```python
from build123d import *

# Parameters (mm, degrees)
SKETCH1_R             = 24.75
SKETCH1_R_2           = 21.75
BOSS_EXTRUDE1_DEPTH   = 90
BOSS_EXTRUDE3_START   = 72
SKETCH5_R             = 29.75
SKETCH5_R_2           = 21.75
BOSS_EXTRUDE3_DEPTH   = 5
SKETCH7_R             = 24.75
SKETCH7_R_2           = 21.75
BOSS_EXTRUDE4_DEPTH   = 2.5
BOSS_EXTRUDE5_START   = -5
SKETCH6_R             = 2
BOSS_EXTRUDE5_DEPTH   = 5
MIRROR2_START         = -92.5
MIRROR2_OUTLINE_R     = 24.75
MIRROR2_OUTLINE_R_2   = 21.75
MIRROR2_DEPTH         = 92.5
MIRROR2_START_2       = 67
MIRROR2_2_OUTLINE_R   = 29.75
MIRROR2_2_OUTLINE_R_2 = 24.75
MIRROR2_2_DEPTH       = 5
MIRROR2_3_OUTLINE_R   = 2
MIRROR2_3_DEPTH       = 5


# Read off the part's stored shape, not the designer's step: Mirror2
with BuildPart() as part:
    # Sketch1 → Boss-Extrude1 (new body)
    with BuildSketch(Plane.XY):
        with Locations(Location((0, 0, 0), (0, 0, 180))):
            Circle(SKETCH1_R)
        with Locations(Location((0, 0, 0), (0, 0, 180))):
            Circle(SKETCH1_R_2, mode=Mode.SUBTRACT)
    extrude(amount=BOSS_EXTRUDE1_DEPTH)

    # Sketch5 → Boss-Extrude3 (add)
    with BuildSketch(Plane.XY.offset(BOSS_EXTRUDE3_START)):
        Circle(SKETCH5_R)
        with Locations(Location((0, 0, 0), (0, 0, 180))):
            Circle(SKETCH5_R_2, mode=Mode.SUBTRACT)
    extrude(amount=BOSS_EXTRUDE3_DEPTH)

    # Sketch7 → Boss-Extrude4 (add, symmetric)
    with BuildSketch(Plane.XY.offset(90)):
        with Locations(Location((0, 0, 0), (0, 0, 180))):
            Circle(SKETCH7_R)
        with Locations(Location((0, 0, 0), (0, 0, 180))):
            Circle(SKETCH7_R_2, mode=Mode.SUBTRACT)
    extrude(amount=BOSS_EXTRUDE4_DEPTH, both=True)

    # Sketch6 → Boss-Extrude5 (add)
    with BuildSketch(Plane.XY.offset(92.5).offset(BOSS_EXTRUDE5_START)):
        with BuildLine():
            Line((-22.997666259, 9.147122314), (-33.267406372, 22.947582732))
            Line((-33.267406372, 22.947582732), (-22.947582732, 33.267406372))
            Line((-22.947582732, 33.267406372), (-9.147122314, 22.997666259))
            ThreePointArc((-9.147122314, 22.997666259), (-17.500892834, 17.500892834), (-22.997666259, 9.147122314))
        make_face()
        with Locations((-20.04683438, 22.097086912)):
            Circle(SKETCH6_R, mode=Mode.SUBTRACT)
        with Locations((-27.04683438, 22.097086912)):
            Circle(SKETCH6_R, mode=Mode.SUBTRACT)
    boss_extrude5 = extrude(amount=BOSS_EXTRUDE5_DEPTH)

    # Mirror1: Boss-Extrude5 across plane
    add(boss_extrude5.mirror(Plane(origin=(0, 0, 0), x_dir=(0, 0, 1), z_dir=(1, 0, 0))))

    # Mirror2 outline → Mirror2 (add)
    with BuildSketch(Plane.XY.offset(MIRROR2_START)):
        Circle(MIRROR2_OUTLINE_R)
        Circle(MIRROR2_OUTLINE_R_2, mode=Mode.SUBTRACT)
    extrude(amount=MIRROR2_DEPTH)

    # Mirror2 2 outline → Mirror2 2 (add)
    with BuildSketch(Plane.XY.offset(MIRROR2_START_2)):
        Circle(MIRROR2_2_OUTLINE_R)
        Circle(MIRROR2_2_OUTLINE_R_2, mode=Mode.SUBTRACT)
    extrude(amount=MIRROR2_2_DEPTH)

    # Mirror2 3 outline → Mirror2 3 (add)
    # profile 1 of 2: a face of its own
    with BuildSketch(Plane.XY.offset(MIRROR2_START)):
        with BuildLine():
            ThreePointArc((9.147122314, 22.997666259), (17.500892834, 17.500892834), (22.997666259, 9.147122314))
            Line((22.997666259, 9.147122314), (33.267406372, 22.947582732))
            Line((33.267406372, 22.947582732), (22.947582732, 33.267406372))
            Line((22.947582732, 33.267406372), (9.147122314, 22.997666259))
        make_face()
        with Locations((20.04683438, 22.097086912)):
            Circle(MIRROR2_3_OUTLINE_R, mode=Mode.SUBTRACT)
        with Locations((27.04683438, 22.097086912)):
            Circle(MIRROR2_3_OUTLINE_R, mode=Mode.SUBTRACT)
    # profile 2 of 2: a face of its own
    with BuildSketch(Plane.XY.offset(MIRROR2_START)):
        with BuildLine():
            ThreePointArc((-22.997666259, 9.147122314), (-17.500892834, 17.500892834), (-9.147122314, 22.997666259))
            Line((-9.147122314, 22.997666259), (-22.947582732, 33.267406372))
            Line((-22.947582732, 33.267406372), (-33.267406372, 22.947582732))
            Line((-33.267406372, 22.947582732), (-22.997666259, 9.147122314))
        make_face()
        with Locations((-20.04683438, 22.097086912)):
            Circle(MIRROR2_3_OUTLINE_R, mode=Mode.SUBTRACT)
        with Locations((-27.04683438, 22.097086912)):
            Circle(MIRROR2_3_OUTLINE_R, mode=Mode.SUBTRACT)
    extrude(amount=MIRROR2_3_DEPTH)


solid = part.part
```
Input: part model. Units: mm. Frame: model coordinates. A direction names the side the tool comes from. Coordinates: 2 decimals unless noted, no trailing zeros. Write each loop counter-clockwise with the first axis right and the second up, starting at its lowest first coordinate (ties: lowest second). Pieces come first, ordered by that corner, then holes. Notation, with made-up numbers: (37.5, -9) -> (52.5, -9) arc R26 cw to (52.5, 15) -> close; hole circle Ø6 at (68.5, 80). An arc over 180 degrees is marked (long way). Answer as a JSON object with one key per item and string values.
1. Section A-A on x = 0. Return the cut outline in (y, z).
Result set:
{"outline": "(-29.75, 67) -> (-24.75, 67) -> (-24.75, -92.5) -> (-21.75, -92.5) -> (-21.75, 92.5) -> (-24.75, 92.5) -> (-24.75, 77) -> (-29.75, 77) -> close; (21.75, -92.5) -> (24.75, -92.5) -> (24.75, 67) -> (29.75, 67) -> (29.75, 77) -> (24.75, 77) -> (24.75, 92.5) -> (21.75, 92.5) -> close"}
2. Section C-C on z = 62. Return the cut outline in (x, y), then the cut area to 3 significant figures.
Result set:
{"outline": "circle Ø49.5 at (0, 0); hole circle Ø43.5 at (0, 0)", "area": "438 mm2"}
3. Mould query, pull axis Y, two halves, no side actions, for faces 5 (the face through (25.05, 22.19, -90.04)), 6 (the face through (-28.18, 28.035, 89.965)), 7 (the face through (24, 21, 87.5)). Classes: released by +Y, released by -Y, zero draft, split by the parting line, or undercut.
Result set:
{"face 5": "undercut", "face 6": "released by +Y", "face 7": "zero draft"}
4. Material intervals for line 1 (Y direction, x = -12.5, z = -34); line 2 (Y direction, x = -11, z = 18); line 3 (X direction, y = 3, z = -80), sorted ascending. Write a range as from..to.
Result set:
{"line 1": "y = -21.36..-17.8, 17.8..21.36", "line 2": "y = -22.17..-18.76, 18.76..22.17", "line 3": "x = -24.57..-21.54, 21.54..24.57"}
5. First-contact query: P1, Ø3, axis at x = 20.05, y = 22.1, coming from the +Z side; P2, Ø3, axis at x = -20.05, y = 22.1, coming from the -Z side; P3, Ø5, axis at y = 7.5, z = -68.5, coming from the -X side. Flat tips, straight axial feed; report the tip coordinate or a pass-through.
Result set:
{"P1": "stops at z = 77", "P2": "stops at z = 67", "P3": "stops at x = -24.24"}
6. Section D-D on x = 16. Return the cut outline in (y, z), then the cut area to 3 significant figures.
Result set:
{"outline": "(-25.08, 67) -> (-18.88, 67) -> (-18.88, -92.5) -> (-14.73, -92.5) -> (-14.73, 92.5) -> (-18.88, 92.5) -> (-18.88, 77) -> (-25.08, 77) -> close; (14.73, -92.5) -> (28.1, -92.5) -> (28.1, -87.5) -> (18.88, -87.5) -> (18.88, 67) -> (25.08, 67) -> (25.08, 77) -> (18.88, 77) -> (18.88, 87.5) -> (28.1, 87.5) -> (28.1, 92.5) -> (14.73, 92.5) -> close", "area": "1,750 mm2"}
7. Access query for faces 1 (the face through (-21.4, 24.1, -87.5)), 2 (the face through (1.6, 24.7, -13.9)), 3 (the face through (-21.634, 20.88, -90.035)), 4 (the face through (-15.95, 28.06, -90.04)). Directions: +Z, -Z, +X, -X, +Y, -Y. A direction counts if a zero-diameter tool reaches every point of the face in a straight line with its end or side. Return the directions, or none.
Result set:
{"face 1": "-X, +Y", "face 2": "none", "face 3": "-Z", "face 4": "-Z, +Y"}
